```python
from build123d import *

# Parameters (mm, degrees)
F0_R     = 12.7
F1_DEPTH = 25.4
F2_DEPTH = 17.78
F3_R     = 5.08
F4_R     = 1.4351
F5_DEPTH = 25.4


with BuildPart() as f1:
    # F0 (on Front) → F1 (new body)
    with BuildSketch(Plane.XZ):
        Circle(F0_R)
    extrude(amount=F1_DEPTH)

    # F0 (on Front) → F2 (join)
    with BuildSketch(Plane.XZ):
        Circle(F0_R)
    extrude(amount=F2_DEPTH)

    # F3
    f3_edges = [f1.edges().sort_by_distance(p)[0] for p in [
        (-12.7, 0, 0),
        (-12.7, -25.4, 0),
    ]]
    fillet(f3_edges, radius=F3_R)

    # F4 (on face) → F5 (cut)
    with BuildSketch(Plane(origin=(0, 0, 0), x_dir=(-1, 0, 0), z_dir=(0, 1, 0))):
        Circle(F4_R)
    extrude(amount=-F5_DEPTH, mode=Mode.SUBTRACT)


solid = f1.part
```
Can you work these out from the model? Positions are in its coordinate system, mm. Coordinates: 2 decimals unless noted, no trailing zeros. Loops run counter-clockwise (first coordinate to the right, second up) from the corner with the lowest first, then second, coordinate; pieces in that order, holes last.
1) For pin 1 (4 mm diameter, centred on x = -8.5, y = -10.5, fed in from +Z); pin 2 (1.5 mm diameter, centred on y = -8.5, z = 8, fed in from -X); pin 3 (8 mm diameter, centred on y = -15, z = -8, fed in from +X), each with a flat end and sliding along its axis, tell me the tip position at first contact or that it passes through.
2) I need wall thicknesses on probe 1 along Z at (x, y) = (0, -12); probe 2 along X at (y, z) = (-8.5, 0.75); probe 3 along Y at (x, z) = (-8.5, -8.5). Which ranges of each line are inside material? Lowest first, please.
3) Imagine slicing it at C-C on y = -6.25. List the corners of the cut face in (x, z) for me.
4) Imagine slicing it at D-D on y = -2. List the corners of the cut face in (x, z) for me.
5) Thinking about a two-plate mould opening in Z: for faces 1 (the cylindrical face through (-2.75, -12.59, -12.4)), 2 (the cylindrical face through (1.14, -12.52, -0.87)), 3 (the flat face through (0, -25.4, -2)), which applies, pulls with the +Z half, pulls with the -Z half, needs draft (parallel to the pull), parting line crosses it, or undercut?
6) Imagine slicing it at A-A on x = 0. List the corners of the cut face in (y, z) for me.
7) Imagine slicing it at B-B on z = 0. List the corners of the cut face in (x, y) for me, plus the area to 3 significant figures.
Completed:
1. pin 1: stops at z = 10.91
1. pin 2: stops at x = -10.43
1. pin 3: stops at x = 12.05
2. probe 1: z = -12.7 to -1.44, 1.44 to 12.7
2. probe 2: x = -12.68 to -1.22, 1.22 to 12.68
2. probe 3: y = -22.86 to -2.54
3. outline: circle Ø25.4 at (0, 0); hole circle Ø2.87 at (0, 0)
4. outline: circle Ø23.32 at (0, 0); hole circle Ø2.87 at (0, 0)
5. face 1: parting line crosses it
5. face 2: undercut
5. face 3: needs draft
6. outline: (-25.4, -7.62) arc R5.08 ccw to (-20.32, -12.7) - (-5.08, -12.7) arc R5.08 ccw to (0, -7.62) - (0, -1.44) - (-25.4, -1.44) - close; (-25.4, 1.44) - (0, 1.44) - (0, 7.62) arc R5.08 ccw to (-5.08, 12.7) - (-20.32, 12.7) arc R5.08 ccw to (-25.4, 7.62) - close
7. outline: (-12.7, -20.32) arc R5.08 ccw to (-7.62, -25.4) - (-1.44, -25.4) - (-1.44, 0) - (-7.62, 0) arc R5.08 ccw to (-12.7, -5.08) - close; (1.44, -25.4) - (7.62, -25.4) arc R5.08 ccw to (12.7, -20.32) - (12.7, -5.08) arc R5.08 ccw to (7.62, 0) - (1.44, 0) - close
7. area: 550 mm2
